from build123d import *

# Parameters (mm, degrees)
F0_R     = 10.95
F1_DEPTH = 3


with BuildPart() as f1:
    # F0 (on Top) → F1 (new body)
    with BuildSketch(Plane.XY):
        with BuildLine():
            ThreePointArc((10.996136, 0.291549), (9.526279, 5.5), (5.750556, 9.377159))
            ThreePointArc((5.750556, 9.377159), (5.5, 9.526279), (5.245579, 9.668707))
            ThreePointArc((5.245579, 9.668707), (0, 11), (-5.245579, 9.668707))
            ThreePointArc((-5.245579, 9.668707), (-5.5, 9.526279), (-5.750556, 9.377159))
            ThreePointArc((-5.750556, 9.377159), (-9.526279, 5.5), (-10.996136, 0.291549))
            ThreePointArc((-10.996136, 0.291549), (-11, 0), (-10.996136, -0.291549))
            ThreePointArc((-10.996136, -0.291549), (-9.526279, -5.5), (-5.750556, -9.377159))
            ThreePointArc((-5.750556, -9.377159), (-5.5, -9.526279), (-5.245579, -9.668707))
            ThreePointArc((-5.245579, -9.668707), (0, -11), (5.245579, -9.668707))
            ThreePointArc((5.245579, -9.668707), (5.5, -9.526279), (5.750556, -9.377159))
            ThreePointArc((5.750556, -9.377159), (9.526279, -5.5), (10.996136, -0.291549))
            ThreePointArc((10.996136, -0.291549), (11, 0), (10.996136, 0.291549))
        make_face()
        with BuildLine():
            ThreePointArc((40.428516, 0), (43.705472, 25.233366), (20.214258, 35.012122))
            ThreePointArc((20.214258, 35.012122), (0, 50.466732), (-20.214258, 35.012122))
            ThreePointArc((-20.214258, 35.012122), (-43.705472, 25.233366), (-40.428516, 0))
            ThreePointArc((-40.428516, 0), (-43.705472, -25.233366), (-20.214258, -35.012122))
            ThreePointArc((-20.214258, -35.012122), (0, -50.466732), (20.214258, -35.012122))
            ThreePointArc((20.214258, -35.012122), (43.705472, -25.233366), (40.428516, 0))
        make_face()
        with Locations((-30.310889, -17.5)):
            Circle(F0_R, mode=Mode.SUBTRACT)
        with Locations((0, -35)):
            Circle(F0_R, mode=Mode.SUBTRACT)
        with BuildLine():
            ThreePointArc((5.245579, 9.668707), (5.5, 9.526279), (5.750556, 9.377159))
            ThreePointArc((5.750556, 9.377159), (9.526279, 5.5), (10.996136, 0.291549))
            ThreePointArc((10.996136, 0.291549), (11, 0), (10.996136, -0.291549))
            ThreePointArc((10.996136, -0.291549), (9.526279, -5.5), (5.750556, -9.377159))
            ThreePointArc((5.750556, -9.377159), (5.5, -9.526279), (5.245579, -9.668707))
            ThreePointArc((5.245579, -9.668707), (0, -11), (-5.245579, -9.668707))
            ThreePointArc((-5.245579, -9.668707), (-5.5, -9.526279), (-5.750556, -9.377159))
            ThreePointArc((-5.750556, -9.377159), (-9.526279, -5.5), (-10.996136, -0.291549))
            ThreePointArc((-10.996136, -0.291549), (-11, 0), (-10.996136, 0.291549))
            ThreePointArc((-10.996136, 0.291549), (-9.526279, 5.5), (-5.750556, 9.377159))
            ThreePointArc((-5.750556, 9.377159), (-5.5, 9.526279), (-5.245579, 9.668707))
            ThreePointArc((-5.245579, 9.668707), (0, 11), (5.245579, 9.668707))
        make_face(mode=Mode.SUBTRACT)
        with Locations((30.310889, -17.5)):
            Circle(F0_R, mode=Mode.SUBTRACT)
        with Locations((-30.310889, 17.5)):
            Circle(F0_R, mode=Mode.SUBTRACT)
        with Locations((30.310889, 17.5)):
            Circle(F0_R, mode=Mode.SUBTRACT)
        with Locations((0, 35)):
            Circle(F0_R, mode=Mode.SUBTRACT)
    extrude(amount=F1_DEPTH)


solid = f1.part
Design review of the part built by this model. Coordinates are the model's own, in mm. A direction names the side the tool comes from. Give positions to 0.01 mm unless a question says otherwise; leave off trailing zeros. Loops run counter-clockwise (first coordinate to the right, second up) from the corner with the lowest first, then second, coordinate; pieces in that order, holes last. Notation, with made-up numbers: (-37, 56) -> (16, 56) arc R12 ccw to (16, 64) -> close; hole circle Ø2 at (-11, -39). An arc over 180 degrees is marked (long way). One line per question, with ' | ' between items. Start each with the question number.
(1) We need section A-A (x = 0). State the section outline as (y, z) points, and give its area (3 significant figures).
(2) Insertion check: P1, Ø10, axis at x = -25, y = -1, coming from the -Z side; P2, Ø17.5, axis at x = 0, y = 35, coming from the +Z side. Each pin has a flat end and moves straight along its axis. Give the tip position at first contact, or say it passes through.
(3) For faces 4 (the face through (0.383, 50.463, 1.479)), 5 (the face through (0, 11, 1)), list the 3-axis set-ups (+Z, -Z, +X, -X, +Y, -Y) from which the entire face can be reached by the end or side of a thin tool; tool diameter is ignored.
(4) We need section B-B (y = 17.5). State the section outline as (x, z) points, and give its area (3 significant figures).
(5) We need section C-C (x = -29.5). State the section outline as (y, z) points, and give its area (3 significant figures).
(6) We need section D-D (y = 41). State the section outline as (x, z) points.
(7) Draft analysis for pull direction Y (two halves, no side actions). For faces 1 (the face through (35.364, 7.785, 1.479)), 2 (the face through (-1, 12, 3)), 3 (the face through (-0.383, -50.463, 1.479)), state which applies: +Y half, -Y half, draft (parallel to the pull), parting line (faces both ways), or undercut.
(8) For line 1 (Y direction, x = 31, z = 2.8); line 2 (X direction, y = 14, z = 1.85); line 3 (Y direction, x = -20.5, z = 0.55), list the stretches that pass through material, from the lowest coordinate up.
The answers:
1) outline: (-50.47, 0) -> (-45.95, 0) -> (-45.95, 3) -> (-50.47, 3) -> close; (-24.05, 0) -> (-11, 0) -> (-11, 3) -> (-24.05, 3) -> close; (11, 0) -> (24.05, 0) -> (24.05, 3) -> (11, 3) -> close; (45.95, 0) -> (50.47, 0) -> (50.47, 3) -> (45.95, 3) -> close | area: 105 mm^2
2) P1: stops at z = 0 | P2: passes through
3) face 4: +Z, -Z, +Y | face 5: +Z, -Z
4) outline: (-46.33, 0) -> (-41.26, 0) -> (-41.26, 3) -> (-46.33, 3) -> close; (-19.36, 0) -> (19.36, 0) -> (19.36, 3) -> (-19.36, 3) -> close; (41.26, 0) -> (46.33, 0) -> (46.33, 3) -> (41.26, 3) -> close | area: 147 mm^2
5) outline: (-35.33, 0) -> (-28.42, 0) -> (-28.42, 3) -> (-35.33, 3) -> close; (-6.58, 0) -> (6.58, 0) -> (6.58, 3) -> (-6.58, 3) -> close; (28.42, 0) -> (35.33, 0) -> (35.33, 3) -> (28.42, 3) -> close | area: 81.0 mm^2
6) outline: (-17.52, 0) -> (-9.16, 0) -> (-9.16, 3) -> (-17.52, 3) -> close; (9.16, 0) -> (17.52, 0) -> (17.52, 3) -> (9.16, 3) -> close
7) face 1: undercut | face 2: draft | face 3: -Y half
8) line 1: y = -34.99 to -28.43, -6.57 to 6.57, 28.43 to 34.99 | line 2: x = -46.5 to -40.69, -19.94 to 19.94, 40.69 to 46.5 | line 3: y = -35.09 to -22.36, -12.64 to 12.64, 22.36 to 35.09
